```python
from build123d import *

# Parameters (mm, degrees)
F0_W     = 180.34
F0_H     = 76.2
F1_DEPTH = 167.64
F2_W     = 50.8
F2_H     = 25.4
F3_DEPTH = 19.05
F4_W     = 1.27
F4_H     = 12.7
F5_DEPTH = 10.16
F7_W     = 76.2
F7_H     = 16.51
F8_DEPTH = 29.23794


with BuildPart() as f1:
    # F0 (on Top) → F1 (new body)
    with BuildSketch(Plane.XY):
        Rectangle(F0_W, F0_H)
    extrude(amount=F1_DEPTH)

    # F2 (on face) → F3 (cut)
    with BuildSketch(Plane.XY.offset(167.64)):
        with Locations((64.77, 25.4)):
            Rectangle(F2_W, F2_H)
        with Locations((-64.77, 25.4)):
            Rectangle(F2_W, F2_H)
    extrude(amount=-F3_DEPTH, mode=Mode.SUBTRACT)

    # F4 (on face) → F5 (join)
    with BuildSketch(Plane.XY.offset(148.59)):
        with Locations((77.47, 24.041014)):
            Rectangle(F4_W, F4_H)
        with Locations((-77.47, 25.339247)):
            Rectangle(F4_W, F4_H)
    extrude(amount=F5_DEPTH)

    # F7 (on face) → F8 (cut)
    with BuildSketch(Plane(origin=(0, 38.1, 0), x_dir=(-1, 0, 0), z_dir=(0, 1, 0))):
        with Locations((0, 158.115)):
            Rectangle(F7_W, F7_H)
    extrude(amount=-F8_DEPTH, mode=Mode.SUBTRACT)


solid = f1.part
```
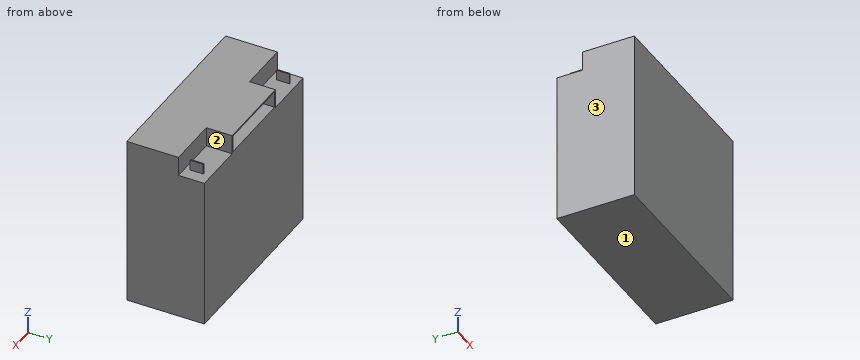
CAD build for the part. Positions are in the model's coordinates, mm. Face numbers are marked on the shaded views. Round coordinates to 2 decimals unless told otherwise and drop trailing zeros. Write each loop counter-clockwise with the first axis right and the second up, starting at its lowest first coordinate (ties: lowest second). Pieces come first, ordered by that corner, then holes. Notation, with made-up numbers: (79, 48) - (126, 48) arc R29 ccw to (126, 69) - close; hole circle Ø1 at (72.5, -31). An arc over 180 degrees is marked (long way). Return JSON: item names as keys, results as strings. Group by question number.
Item 1: Band-saw the part on B-B on x = 60.5. List the corners of the cut face in (y, z), plus the area to 3 significant figures.
Item 2: Probe probe 1 along Z at (x, y) = (-20, 25); probe 2 along Y at (x, z) = (81.5, 154.5); probe 3 along Z at (x, y) = (42.5, 20). List the from-to ranges inside material, lowest first.
Item 3: Band-saw the part on C-C on x = -5. List the corners of the cut face in (y, z), plus the area to 3 significant figures.
Item 4: Flat gauge pins, fed straight in: pin 1 Ø3 at (x, y) = (-72, 24.5) entering from +Z; pin 2 Ø8 at (y, z) = (24, 153.5) entering from -X (3 decimals); pin 3 Ø8 at (y, z) = (23.5, 154) entering from +X (3 decimals). Where does each tip first touch, or does it go through?
Item 5: Band-saw the part on A-A on y = 21.5. List the corners of the cut face in (x, z) (3 decimals), plus the area to 3 significant figures.
Item 6: Mould opens along X. For the marked faces 1, 2 and 3 say: +X half, -X half, draft (parallel to the pull), parting line (faces both ways), or undercut.
Resolved:
{
 "1": {"outline": "(-38.1, 0) - (38.1, 0) - (38.1, 148.59) - (12.7, 148.59) - (12.7, 167.64) - (-38.1, 167.64) - close", "area": "12,300 mm²"},
 "2": {"probe 1": "z = 0 to 149.86, 166.37 to 167.64", "probe 2": "y = -38.1 to 12.7", "probe 3": "z = 0 to 148.59"},
 "3": {"outline": "(-38.1, 0) - (38.1, 0) - (38.1, 149.86) - (8.86, 149.86) - (8.86, 166.37) - (38.1, 166.37) - (38.1, 167.64) - (-38.1, 167.64) - close", "area": "12,300 mm²"},
 "4": {"pin 1": "stops at z = 148.59", "pin 2": "stops at x = -78.105", "pin 3": "stops at x = 78.105"},
 "5": {"outline": "(-90.17, 0) - (90.17, 0) - (90.17, 148.59) - (78.105, 148.59) - (78.105, 158.75) - (76.835, 158.75) - (76.835, 148.59) - (39.37, 148.59) - (39.37, 167.64) - (-39.37, 167.64) - (-39.37, 148.59) - (-76.835, 148.59) - (-76.835, 158.75) - (-78.105, 158.75) - (-78.105, 148.59) - (-90.17, 148.59) - close; hole (-38.1, 149.86) - (38.1, 149.86) - (38.1, 166.37) - (-38.1, 166.37) - close", "area": "27,100 mm²"},
 "6": {"face 1": "draft", "face 2": "undercut", "face 3": "-X half"}
}
